```python
from build123d import *

# Parameters (mm, degrees)
SKETCH1_W           = 193.68
SKETCH1_H           = 190.5
BOSS_EXTRUDE1_DEPTH = 4.78
SKETCH2_R           = 2.286
CUT_EXTRUDE1_DEPTH  = 5.78
CUT_EXTRUDE2_DEPTH  = 5.78
SKETCH4_R           = 1.3
CUT_EXTRUDE4_DEPTH  = 5.78


with BuildPart() as part:
    # Sketch1 → Boss-Extrude1 (new body)
    with BuildSketch(Plane(origin=(0, 0, 0), x_dir=(1, 0, 0), z_dir=(0, 1, 0))):
        Rectangle(SKETCH1_W, SKETCH1_H)
    extrude(amount=BOSS_EXTRUDE1_DEPTH)

    # Sketch2 → Cut-Extrude1 (cut, through all)
    with BuildSketch(Plane(origin=(0, 4.78, 0), x_dir=(1, 0, 0), z_dir=(0, 1, 0))):
        with Locations((0, 82.55)):
            Circle(SKETCH2_R)
    extrude(amount=-CUT_EXTRUDE1_DEPTH, mode=Mode.SUBTRACT)

    # Sketch3 → Cut-Extrude2 (cut, through all)
    with BuildSketch(Plane(origin=(0, 4.78, 0), x_dir=(1, 0, 0), z_dir=(0, 1, 0))):
        Polygon((0, -95.25), (-32.28, -95.25), (-32.28, -70.249999962), (32.28, -70.249999962), (32.28, -95.25), align=None)
    extrude(amount=-CUT_EXTRUDE2_DEPTH, mode=Mode.SUBTRACT)

    # Sketch4 → Cut-Extrude4 (cut, through all)
    with BuildSketch(Plane(origin=(0, 4.78, 0), x_dir=(1, 0, 0), z_dir=(0, 1, 0))):
        with Locations((-30.511, -56.699999962)):
            Circle(SKETCH4_R)
        with Locations((30.289, -56.699999962)):
            Circle(SKETCH4_R)
    extrude(amount=-CUT_EXTRUDE4_DEPTH, mode=Mode.SUBTRACT)


solid = part.part
```
The model under review builds one solid part; all positions refer to its coordinate system, in mm. A direction names the side the tool comes from. Coordinates: 2 decimals unless noted, no trailing zeros. Loops run counter-clockwise (first coordinate to the right, second up) from the corner with the lowest first, then second, coordinate; pieces in that order, holes last. Notation, with made-up numbers: (75.5, 86) -> (79.5, 86) arc R20 cw to (79.5, 124) -> close; hole circle Ø4 at (-40, 17). An arc over 180 degrees is marked (long way). Answer as CSV lines item,"result".
Item 1: Draft analysis for pull direction X (two halves, no side actions). For faces 3 (the flat face through (-65, 2, 95.25)), 4 (the cylindrical face through (-0.298, 2.423, -84.817)), 5 (the flat face through (96.84, 2, 1)), state which applies: +X half, -X half, draft (parallel to the pull), parting line (faces both ways), or undercut.
Results below:
face 3,"draft"
face 4,"undercut"
face 5,"+X half"
Item 2: For L1, parallel to X at y = 1.65, z = 56.7; L2, parallel to X at y = 3, z = -82.55; L3, parallel to Z at x = 0, y = 1.85, list the stretches that pass through material, from the lowest coordinate up.
Results below:
L1,"x = -96.84 to -31.81, -29.21 to 28.99, 31.59 to 96.84"
L2,"x = -96.84 to -2.29, 2.29 to 96.84"
L3,"z = -95.25 to -84.84, -80.26 to 70.25"
Item 3: Take a section at C-C, the plane y = 3.25. State the section outline as (x, z) points.
Results below:
outline,"(-96.84, -95.25) -> (96.84, -95.25) -> (96.84, 95.25) -> (32.28, 95.25) -> (32.28, 70.25) -> (-32.28, 70.25) -> (-32.28, 95.25) -> (-96.84, 95.25) -> close; hole circle Ø2.6 at (-30.51, 56.7); hole circle Ø4.57 at (0, -82.55); hole circle Ø2.6 at (30.29, 56.7)"
Item 4: Take a section at B-B, the plane x = 0. State the section outline as (y, z) points, and give its area (3 significant figures).
Results below:
outline,"(0, -95.25) -> (4.78, -95.25) -> (4.78, -84.84) -> (0, -84.84) -> close; (0, -80.26) -> (4.78, -80.26) -> (4.78, 70.25) -> (0, 70.25) -> close"
area,"769 mm2"
Item 5: Take a section at D-D, the plane x = -20. State the section outline as (y, z) points, and give its area (3 significant figures).
Results below:
outline,"(0, -95.25) -> (4.78, -95.25) -> (4.78, 70.25) -> (0, 70.25) -> close"
area,"791 mm2"
Item 6: Machinability: for faces 1 (the flat face through (-1, 0, -1)), 2 (the flat face through (32.28, 2, 83)), which of the approach directions +Z, -Z, +X, -X, +Y, -Y give a long, thin tool a straight path to every point of the face, cutting with its end or side? Answer none if there is none.
Results below:
face 1,"+Z, -Z, +X, -X, -Y"
face 2,"+Z, +Y, -Y"
Item 7: Take a section at A-A, the plane z = -82.55. State the section outline as (x, y) points, and give its area (3 significant figures).
Results below:
outline,"(-96.84, 0) -> (-2.29, 0) -> (-2.29, 4.78) -> (-96.84, 4.78) -> close; (2.29, 0) -> (96.84, 0) -> (96.84, 4.78) -> (2.29, 4.78) -> close"
area,"904 mm2"
Item 8: Insertion check: pin 1 (2.5 mm diameter, centred on x = -9.5, y = 3, fed in from +Z). The pin has a flat end and moves straight along its axis. Give the tip position at first contact, or say it passes through.
Results below:
pin 1,"stops at z = 70.25"
